Build history of the part. All positions in model axes, mm. A direction names the side the tool comes from. Give positions to 0.01 mm unless a question says otherwise; leave off trailing zeros. Write each loop counter-clockwise with the first axis right and the second up, starting at its lowest first coordinate (ties: lowest second). Pieces come first, ordered by that corner, then holes. Notation, with made-up numbers: (-2, 86.25) -> (42, 86.25) arc R18 ccw to (42, 107.25) -> close; hole circle Ø6 at (-14.75, -33). An arc over 180 degrees is marked (long way). One line per question, with ' | ' between items. Start each with the question number.
(1) Drill centre lines: probe 1 along Y at (x, z) = (0, -1); probe 2 along Y at (x, z) = (-2.5, 4); probe 3 along X at (y, z) = (4.5, -22). Where is each one in solid material? Low to high. Write a range as from..to.
(2) Band-saw the part on C-C, the plane z = -5. Give the cut face in (x, y).
(3) Band-saw the part on A-A, the plane x = 0. Give the cut face in (y, z) (3 decimals).
(4) Band-saw the part on D-D, the plane z = 0.5. Give the cut face in (x, y).
(5) Pin check, flat tips, straight feed: P1, Ø3, axis at x = -10, z = -5, coming from the +Y side; P2, Ø2.5, axis at x = -0.5, y = 6, coming from the +Z side; P3, Ø4, axis at x = 1, y = 1, coming from the -Z side; P4, Ø3.5, axis at x = -7, y = 8, coming from the +Z side. Stop position of each tip, or through.
(6) Tool access for faces 1 (the flat face through (5.2, 0.1, -30)), 2 (the flat face through (-0.01, 11.28, 7.74)), 3 (the flat face through (-2, 8, 0)): list every direction of +Z, -Z, +X, -X, +Y, -Y with a clear straight run to the whole face (end or side of a thin tool).
(7) Band-saw the part on B-B, the plane y = 0. Give the cut face in (x, z) (3 decimals).
from build123d import *

# Parameters (mm, degrees)
F0_R             = 8
F1_DEPTH         = 30
F2_R             = 12.75
F3_DEPTH         = 10
F4_SIZE2         = 6
F4_SIZE          = 2
F7_R             = 2
F8_R             = 5
F9_DEPTH         = 39
F11_DEPTH        = 28.5
F13_DEPTH        = 0.5
F13_COPIES_COUNT = 12
F15_DEPTH        = 1


# Not quite as in the source:
# - a pattern or mirror of a feature is missing from the dataset's text; its kind, count and spacing are read off the source's solid


with BuildPart() as f1:
    # F0 (on Top) → F1 (new body)
    with BuildSketch(Plane.XY):
        Circle(F0_R)
    extrude(amount=-F1_DEPTH)

    # F2 (on Top) → F3 (join)
    with BuildSketch(Plane.XY):
        Circle(F2_R)
    extrude(amount=F3_DEPTH)

    # F4
    f4_edges = [f1.edges().sort_by_distance(p)[0] for p in [
        (-12.75, 0, 10),
    ]]
    f4_side = f1.faces().sort_by_distance((0, 0, 10))[0]
    chamfer(f4_edges, length=F4_SIZE, length2=F4_SIZE2, reference=f4_side)

    # F5 (on Front) → F6 (revolve)
    with BuildSketch(Plane.XZ):
        with BuildLine():
            Line((0, 10), (10.5, 10))
            ThreePointArc((10.5, 10), (5.2737557774, 10.749435663), (0, 11))
            Line((0, 11), (0, 10))
        make_face()
    revolve(axis=Axis((0, 0, 11.4106573164), (0, 0, -1)))

    # F7
    f7_edges = [f1.edges().sort_by_distance(p)[0] for p in [
        (-12.75, 0, 0),
    ]]
    fillet(f7_edges, radius=F7_R)

    # F8 (on face) → F9 (cut)
    with BuildSketch(Plane(origin=(0, 0, -30), x_dir=(1, 0, 0), z_dir=(0, 0, -1))):
        Circle(F8_R)
    extrude(amount=-F9_DEPTH, mode=Mode.SUBTRACT)

    # F10 (on face) → F11 (join)
    with BuildSketch(Plane(origin=(0, 0, 9), x_dir=(1, 0, 0), z_dir=(0, 0, -1))):
        Polygon((0, 6), (-4.867254519, 3), (5.0389095293, 3), align=None)
    extrude(amount=F11_DEPTH)

    # F12 (on Front) → F13 (cut, symmetric)
    with BuildSketch(Plane.XZ):
        Polygon((-13.3409490809, 2.9869333375), (-9.9859265611, 10.7209142298), (-13.1098602818, 12.8878117818), (-16.7612417104, 4.4706658365), align=None)
    f13 = extrude(amount=F13_DEPTH, both=True, mode=Mode.SUBTRACT)

    # F13_copies: F13 ×12 about axis
    f13_copies_axis = Axis((0, 0, 0), (0, 0, 1))
    for i in range(1, F13_COPIES_COUNT):
        add(f13.rotate(f13_copies_axis, i * 360 / F13_COPIES_COUNT), mode=Mode.SUBTRACT)

    # F14 (on face) → F15 (cut)
    with BuildSketch(Plane.XY.offset(10)):
        Polygon((1.9268689083, 4.5769295732), (1.9268689083, 6.5769295732), (-1.8981318941, 6.5769295732), (-1.8981318941, 7.2769295732), (-4.6231322793, 5.3769295732), (-1.8981318941, 3.8769295732), (-1.8981318941, 4.5769295732), align=None)
    extrude(amount=F15_DEPTH, mode=Mode.SUBTRACT)


solid = f1.part
Results:
1) probe 1: y = -8..-3, 5..8 | probe 2: y = -12.5..-3, 4.33..12.5 | probe 3: x = -6.61..-2.18, 2.18..6.61
2) outline: circle Ø16 at (0, 0); hole (-4, -3) -> (4, -3) arc R5 ccw (long way) to start
3) outline: (-12.75, 2) arc R2 ccw to (-10.75, 0) -> (-8, 0) -> (-8, -30) -> (-5, -30) -> (-5, -19.5) -> (-3, -19.5) -> (-3, 9) -> (5, 9) -> (5, -30) -> (8, -30) -> (8, 0) -> (10.75, 0) arc R2 ccw to (12.75, 2) -> (12.75, 4) -> (12.247, 5.508) -> (10.281, 10.042) arc R55.625 ccw to (6.577, 10.61) -> (6.577, 10) -> (4.577, 10) -> (4.577, 10.811) arc R55.625 ccw to (-10.281, 10.042) -> (-12.247, 5.508) -> (-12.75, 4) -> close
4) outline: circle Ø24.15 at (0, 0); hole (-4, -3) -> (4, -3) arc R5 ccw (long way) to start
5) P1: passes through | P2: stops at z = 10.61 | P3: stops at z = 9 | P4: stops at z = 10.29
6) face 1: -Z, +X, -X, +Y, -Y | face 2: +Z, +Y | face 3: -Z
7) outline: (-12.75, 2) arc R2 ccw to (-10.75, 0) -> (-8, 0) -> (-8, -30) -> (-5, -30) -> (-5, 9) -> (5, 9) -> (5, -30) -> (8, -30) -> (8, 0) -> (10.75, 0) arc R2 ccw to (12.75, 2) -> (12.75, 4) -> (12.247, 5.508) -> (10.281, 10.042) arc R55.625 ccw to (-10.281, 10.042) -> (-12.247, 5.508) -> (-12.75, 4) -> close
